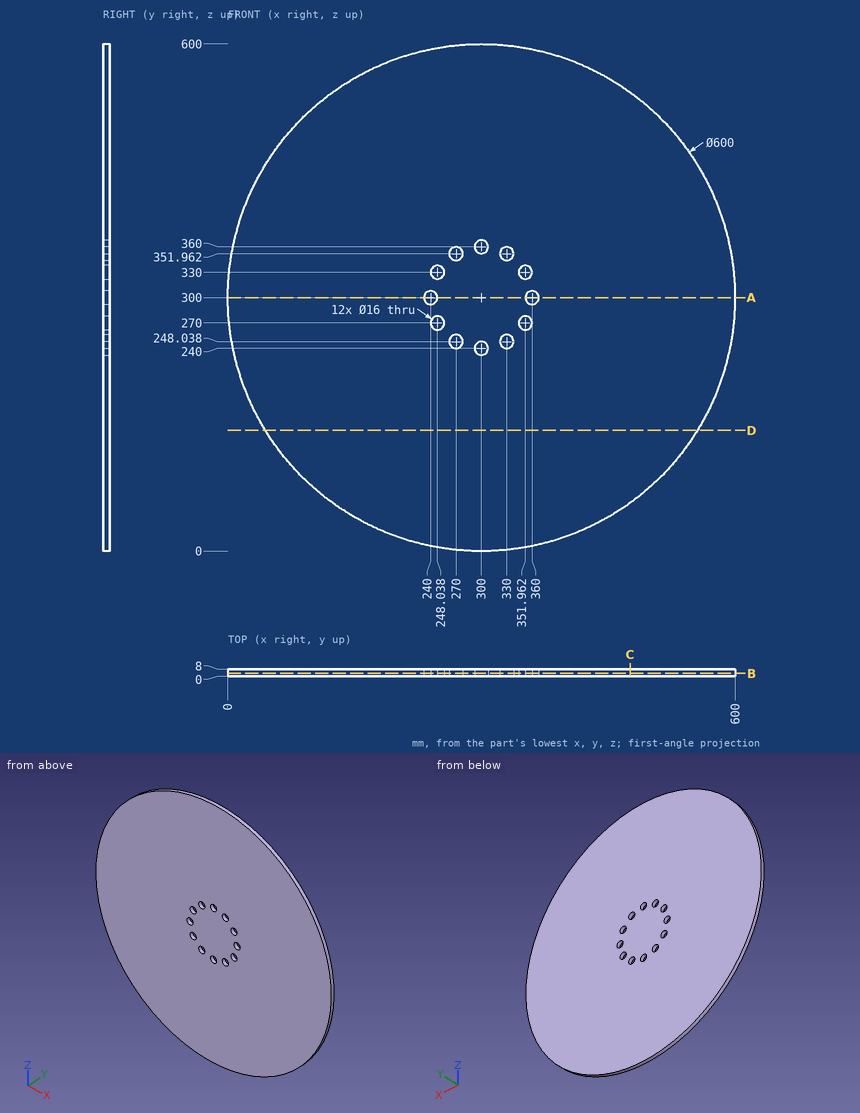
Could you check a few things on this drawing? It's one solid part, dimensions in mm from its lowest x, y, z. Round coordinates to 2 decimals unless told otherwise and drop trailing zeros. Order: outer loops, then holes, each group sorted by start corner. A loop starts at its lowest first (then second) coordinate and runs counter-clockwise, first axis right, second up.
Q1. I'm going to push flat-ended pins straight in: P1, Ø2, axis at x = 79, y = 5.5, coming from the +Z side; P2, Ø14.5, axis at x = 360, z = 300, coming from the +Y side; P3, Ø1, axis at x = 84.5, y = 4, coming from the -Z side (1 decimal); P4, Ø2, axis at y = 6, z = 417.5, coming from the +X side (1 decimal). Where does each tip first touch, or does it pass through?
Geometry says:
P1: stops at z = 503.96
P2: passes through
P3: stops at z = 90.8
P4: stops at x = 576.5
Q2. Imagine slicing it at A-A, the plane z = 300. List the corners of the cut face in (x, y) for me.
Geometry says:
outline: (0, 0) - (232, 0) - (232, 8) - (0, 8) - close; (248, 0) - (352, 0) - (352, 8) - (248, 8) - close; (368, 0) - (600, 0) - (600, 8) - (368, 8) - close
Q3. Imagine slicing it at B-B, the plane y = 3. State how many separate pieces and enclosed holes the cut face has, then the cut area to 3 significant figures.
Geometry says:
separate pieces: 1
enclosed holes: 12
area: 280,000 mm2
Q4. Imagine slicing it at C-C, the plane x = 476. List the corners of the cut face in (y, z) for me, then the cut area to 3 significant figures.
Geometry says:
outline: (0, 57.05) - (8, 57.05) - (8, 542.95) - (0, 542.95) - close
area: 3,890 mm2
Q5. Imagine slicing it at D-D, the plane z = 143. List the corners of the cut face in (x, y) for me, then the cut area to 3 significant figures.
Geometry says:
outline: (44.36, 0) - (555.64, 0) - (555.64, 8) - (44.36, 8) - close
area: 4,090 mm2
Q6. Please list where these lines run through material, in increasing order: probe 1 along X at (y, z) = (2, 300); probe 2 along X at (y, z) = (4.25, 270); probe 3 along Z at (x, y) = (325.5, 7.25) (1 decimal).
Geometry says:
probe 1: x = 0 to 232, 248 to 352, 368 to 600
probe 2: x = 1.5 to 240.04, 256.04 to 343.96, 359.96 to 598.5
probe 3: z = 1.1 to 241.4, 254.7 to 345.3, 358.6 to 598.9
